```python
from build123d import *

# Parameters (mm, degrees)
SKETCH1_R           = 5
BOSS_EXTRUDE1_DEPTH = 30
SKETCH2_W           = 25
SKETCH2_H           = 10
SKETCH2_H_2         = 22
CUT_EXTRUDE1_DEPTH  = 77.962109955


with BuildPart() as part:
    # Sketch1 → Boss-Extrude1 (new body)
    with BuildSketch(Plane.XY):
        with BuildLine():
            Line((0, 10), (57.993870082, 10))
            ThreePointArc((57.993870082, 10), (67.993870082, 0), (57.993870082, -10))
            Line((57.993870082, -10), (0, -10))
            ThreePointArc((0, -10), (-10, 0), (0, 10))
        make_face()
        Circle(SKETCH1_R, mode=Mode.SUBTRACT)
        with Locations((57.993870082, 0)):
            Circle(SKETCH1_R, mode=Mode.SUBTRACT)
    extrude(amount=BOSS_EXTRUDE1_DEPTH)

    # Sketch2 → Cut-Extrude1 (cut, through all)
    with BuildSketch(Plane(origin=(0, 10, 0), x_dir=(1, 0, 0), z_dir=(0, 1, 0))):
        with Locations((2.5, -15)):
            Rectangle(SKETCH2_W, SKETCH2_H)
        with Locations((55.493870082, -15)):
            Rectangle(SKETCH2_W, SKETCH2_H_2)
    extrude(amount=-CUT_EXTRUDE1_DEPTH, mode=Mode.SUBTRACT)


solid = part.part
```
Part model, mm, in its own coordinate system. A direction names the side the tool comes from. Round coordinates to 2 decimals unless told otherwise and drop trailing zeros. Order: outer loops, then holes, each group sorted by start corner. A loop starts at its lowest first (then second) coordinate and runs counter-clockwise, first axis right, second up. Notation, with made-up numbers: M 2,41 L 58,41 A7 cw 58,48 Z; hole C 67.5,71 d1. An arc over 180 degrees is marked long. Put each result on its own line as item: value. Start each with the question number.
1. Tool access for faces 1 (the face through (52.5, 0.1, 4)), 2 (the face through (67.99, 0.22, 27.97)), 3 (the face through (5, 2, 20)): list every direction of +Z, -Z, +X, -X, +Y, -Y with a clear straight run to the whole face (end or side of a thin tool).
2. Slice it at B-B on x = 47.5. List the corners of the cut face in (y, z).
3. Slice it at D-D on z = 28.25. List the corners of the cut face in (x, y).
4. Drop flat-ended pins along their axis: pin 1 (6 mm diameter, centred on x = 0, y = 0, fed in from -Z); pin 2 (1.5 mm diameter, centred on y = -5, z = 6, fed in from +X); pin 3 (3 mm diameter, centred on y = 4, z = 13, fed in from -X). Give the stop position or say it passes through.
5. Slice it at C-C on z = 22.75. List the corners of the cut face in (x, y).
6. Drill centre lines: probe 1 along X at (y, z) = (0, 28.55); probe 2 along X at (y, z) = (0, 23.5); probe 3 along Z at (x, y) = (52, 0.75). Where is each one in solid material? Low to high. Write a range as [from, to].
7. Slice it at A-A on y = 0. List the corners of the cut face in (x, z).
8. Two-plate mould, pull along Z, no slides. Class faces 4 (the face through (5, 2, 10)), 5 (the face through (30, 0, 0)), 6 (the face through (30, 0, 30)), 7 (the face through (62.61, -1.92, 1.97)): +Z half, -Z half, draft (parallel to the pull), parting line (faces both ways), or undercut.
Findings:
1. face 1: +X, +Y, -Y
1. face 2: +Z, -Z, +X
1. face 3: -X, +Y, -Y
2. outline: M -10,0 L 10,0 L 10,4 L -10,4 Z; M -10,26 L 10,26 L 10,30 L -10,30 Z
3. outline: M 0,-10 L 57.99,-10 A10 ccw 57.99,10 L 0,10 A10 ccw Z; hole C 0,0 d10; hole C 57.99,0 d10
4. pin 1: through
4. pin 2: x = 42.99
4. pin 3: x = 15
5. outline: M 0,-10 L 42.99,-10 L 42.99,10 L 0,10 A10 ccw Z; hole C 0,0 d10
6. probe 1: [-10, -5], [5, 52.99], [62.99, 67.99]
6. probe 2: [-10, -5], [5, 42.99]
6. probe 3: [0, 4], [26, 30]
7. outline: M -10,0 L -5,0 L -5,10 L -10,10 Z; M -10,20 L -5,20 L -5,30 L -10,30 Z; M 5,0 L 52.99,0 L 52.99,4 L 42.99,4 L 42.99,26 L 52.99,26 L 52.99,30 L 5,30 L 5,20 L 15,20 L 15,10 L 5,10 Z; M 62.99,0 L 67.99,0 L 67.99,4 L 62.99,4 Z; M 62.99,26 L 67.99,26 L 67.99,30 L 62.99,30 Z
8. face 4: undercut
8. face 5: -Z half
8. face 6: +Z half
8. face 7: draft
